The drawing under review shows one solid part. Ordinate dimensions are in mm from its lowest x, y, z. Give positions to 0.01 mm unless a question says otherwise; leave off trailing zeros. Write each loop counter-clockwise with the first axis right and the second up, starting at its lowest first coordinate (ties: lowest second). Pieces come first, ordered by that corner, then holes. Notation, with made-up numbers: M 48,37.5 L 84,37.5 A26 cw 84,53.5 Z; hole C 79.5,-12 d7. An arc over 180 degrees is marked long. Answer as a JSON object with one key per item and string values. Group by question number.
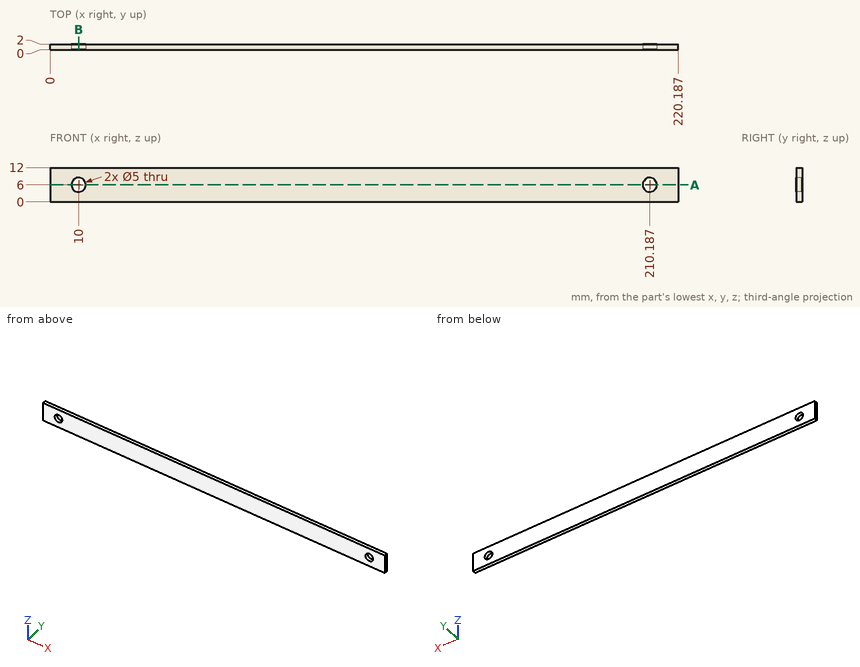
Item 1: Consider section A-A (z = 6). Give the boundary of the cut face in (x, y).
Item 2: To check wall thickness, follow probe 1 along X at (y, z) = (1.75, 7); probe 2 along Z at (x, y) = (10, 1); probe 3 along X at (y, z) = (1.15, 8.25) (1 decimal). State the ranges of each line that lie inside material, in increasing order.
Item 3: Consider section B-B (x = 10). Give the boundary of the cut face in (y, z).
Item 4: Insertion check: P1, Ø4.5, axis at x = 10, z = 6, coming from the -Y side. The pin has a flat end and moves straight along its axis. Give the tip position at first contact, or say it passes through.
Result set:
{
 "1": {"outline": "M 0,0 L 7.5,0 L 7.5,2 L 0,2 Z; M 12.5,0 L 207.69,0 L 207.69,2 L 12.5,2 Z; M 212.69,0 L 220.19,0 L 220.19,2 L 212.69,2 Z"},
 "2": {"probe 1": "x = 0 to 7.71, 12.29 to 207.9, 212.48 to 220.19", "probe 2": "z = 0 to 3.5, 8.5 to 12", "probe 3": "x = 0 to 8.9, 11.1 to 209.1, 211.3 to 220.2"},
 "3": {"outline": "M 0,0 L 2,0 L 2,3.5 L 0,3.5 Z; M 0,8.5 L 2,8.5 L 2,12 L 0,12 Z"},
 "4": {"P1": "passes through"}
}
